from build123d import *

# Parameters (mm, degrees)
SKETCH2_W           = 304.8
SKETCH2_H           = 304.8
BOSS_EXTRUDE1_DEPTH = 15
SKETCH2_3_W         = 57
SKETCH2_3_H         = 3
SKETCH2_3_W_2       = 93.5
SKETCH2_3_W_3       = 130
SKETCH2_3_W_4       = 3
SKETCH2_3_H_2       = 16
SKETCH2_3_H_3       = 17.5
BOSS_EXTRUDE2_DEPTH = 17.5
CUT_EXTRUDE1_DEPTH  = 17.5
CUT_EXTRUDE2_DEPTH  = 17.5
CUT_EXTRUDE3_DEPTH  = 17.5
CUT_EXTRUDE4_DEPTH  = 17.5
CUT_EXTRUDE5_DEPTH  = 17.5
SKETCH2_5_R         = 2
BOSS_EXTRUDE3_DEPTH = 20
SKETCH8_W           = 20
SKETCH8_H           = 95
BOSS_EXTRUDE4_DEPTH = 45
CUT_EXTRUDE6_DEPTH  = 45
SKETCH11_W          = 12.681432754
SKETCH11_H          = 17.5
CUT_EXTRUDE8_DEPTH  = 35
SKETCH10_R          = 2
CUT_EXTRUDE7_DEPTH  = 45


with BuildPart() as part:
    # Sketch2 → Boss-Extrude1 (new body)
    with BuildSketch(Plane.XY):
        with Locations((152.4, 152.4)):
            Rectangle(SKETCH2_W, SKETCH2_H)
    extrude(amount=-BOSS_EXTRUDE1_DEPTH)

    # Sketch2_3 → Boss-Extrude2 (add)
    with BuildSketch(Plane.XY):
        Polygon((93.5, 282.8), (0, 282.8), (0, 279.8), (21.107831574, 279.8), (24.107831574, 279.8), (93.5, 279.8), align=None)
        with BuildLine():
            Line((40, 256.8), (40, 259.8))
            ThreePointArc((40, 259.8), (16.665476221, 250.134523779), (7, 226.8))
            Line((7, 226.8), (7, 180.8))
            Line((7, 180.8), (10, 180.8))
            Line((10, 180.8), (10, 226.8))
            ThreePointArc((10, 226.8), (18.786796564, 248.013203436), (40, 256.8))
        make_face()
        with Locations((65, 238.3)):
            Rectangle(SKETCH2_3_W, SKETCH2_3_H)
        with BuildLine():
            ThreePointArc((93.5, 302.8), (126.5, 269.8), (93.5, 236.8))
            Line((93.5, 236.8), (93.5, 239.8))
            ThreePointArc((93.5, 239.8), (123.5, 269.8), (93.5, 299.8))
            Line((93.5, 299.8), (93.5, 302.8))
        make_face()
        with Locations((46.75, 301.3)):
            Rectangle(SKETCH2_3_W_2, SKETCH2_3_H)
        with BuildLine():
            Line((7, 180.8), (10, 180.8))
            ThreePointArc((10, 180.8), (21.719007055, 152.507814231), (50.011192824, 140.788807176))
            Line((50.011192824, 140.788807176), (50.011192824, 137.788807176))
            ThreePointArc((50.011192824, 137.788807176), (19.597686711, 150.386493887), (7, 180.8))
        make_face()
        with Locations((115.011192824, 139.288807176)):
            Rectangle(SKETCH2_3_W_3, SKETCH2_3_H)
        with BuildLine():
            Line((180.011192824, 140.788807176), (180.011192824, 137.788807176))
            ThreePointArc((180.011192824, 137.788807176), (225.294551046, 153.531340693), (251.047093253, 193.969150516))
            Line((251.047093253, 193.969150516), (248.127809674, 194.660369283))
            ThreePointArc((248.127809674, 194.660369283), (223.433591119, 155.884387261), (180.011192824, 140.788807176))
        make_face()
        Polygon((252.275122275, 212.176070758), (255.194405854, 211.484851991), (251.047093253, 193.969150516), (248.127809674, 194.660369283), align=None)
        with BuildLine():
            ThreePointArc((281.424928951, 191.366981998), (283.869077464, 188.002900174), (284.733622888, 183.935533743))
            Line((284.733622888, 183.935533743), (284.733622888, 151.387820597))
            Line((284.733622888, 151.387820597), (281.733622888, 151.387820597))
            Line((281.733622888, 151.387820597), (281.733622888, 182.599847688))
            ThreePointArc((281.733622888, 182.599847688), (280.869077464, 186.667214118), (278.424928951, 190.031295942))
            Line((278.424928951, 190.031295942), (258.945596653, 207.570565524))
            Line((258.945596653, 207.570565524), (260.952988472, 209.8))
            Line((260.952988472, 209.8), (281.424928951, 191.366981998))
        make_face()
        Polygon((304.8, 124.8), (304.8, 279.8), (301.8, 279.8), (301.8, 148.186252327), (301.8, 133.38760374), (301.8, 124.8), align=None)
        with BuildLine():
            Line((301.8, 133.38760374), (301.8, 148.186252327))
            ThreePointArc((301.8, 148.186252327), (295.901436431, 128.741294171), (280.193920133, 115.850468689))
            Line((280.193920133, 115.850468689), (293.866088671, 121.513666325))
            ThreePointArc((293.866088671, 121.513666325), (298.395845267, 127.074583472), (301.8, 133.38760374))
        make_face()
        Polygon((287.505261485, 115.631748836), (304.8, 122.795464086), (304.8, 124.8), (301.8, 124.8), (293.866088671, 121.513666325), (280.193920133, 115.850468689), (257.453782439, 106.431195246), (260.952988472, 104.633437242), (284.733622888, 114.483698539), align=None)
        Polygon((263.8, 20), (263.8, 0), (304.8, 0), (304.8, 33), (301.8, 33), (301.8, 3), (266.8, 3), (266.8, 20), align=None)
        Polygon((91.199667441, 27.530149764), (92.438635381, 24.873174442), (89.266558126, 23.394010526), (86.547634765, 22.126155741), (83.375557511, 20.646991825), (82.126335472, 23.374526297), align=None)
        with Locations((22.607831574, 271.8)):
            Rectangle(SKETCH2_3_W_4, SKETCH2_3_H_2)
        with Locations((47.84178582, 228.05)):
            Rectangle(SKETCH2_3_W_4, SKETCH2_3_H_3)
        with Locations((114.353619172, 129.788807176)):
            Rectangle(SKETCH2_3_W_4, SKETCH2_3_H_2)
        Polygon((294.010879835, 99.925796783), (287.505261485, 115.631748836), (284.733622888, 114.483698539), (291.239241238, 98.777746486), align=None)
        Polygon((10.107831574, 4.345500571), (5, 16.3), (16, 21), (21.107831574, 9.045500571), align=None)
        Polygon((97.718923361, 5.267854785), (95, 4), (86.547634765, 22.126155741), (89.266558126, 23.394010526), align=None)
    extrude(amount=BOSS_EXTRUDE2_DEPTH)

    # Sketch3 → Cut-Extrude1 (cut)
    with BuildSketch(Plane(origin=(79.564500346, 37.101535829, 0), x_dir=(0, 0, 1), z_dir=(-0.906307787, -0.422618262, 0))):
        Polygon((17.5, -16.523503717), (0, -36.523503717), (17.5, -36.523503717), align=None)
    extrude(amount=-CUT_EXTRUDE1_DEPTH, mode=Mode.SUBTRACT)

    # Sketch4 → Cut-Extrude2 (cut)
    with BuildSketch(Plane(origin=(283.511449018, 117.434287271, 0), x_dir=(0, 0, 1), z_dir=(-0.923879533, -0.382683432, 0))):
        Polygon((17.5, -3.452640544), (0, -20.19369423), (17.5, -20.19369423), align=None)
    extrude(amount=-CUT_EXTRUDE2_DEPTH, mode=Mode.SUBTRACT)

    # Sketch5 → Cut-Extrude3 (cut)
    with BuildSketch(Plane.ZY.offset(-112.853619172)):
        Polygon((17.5, 137.788807176), (17.5, 121.788807176), (0, 121.788807176), align=None)
    extrude(amount=-CUT_EXTRUDE3_DEPTH, mode=Mode.SUBTRACT)

    # Sketch6 → Cut-Extrude4 (cut)
    with BuildSketch(Plane.ZY.offset(-46.34178582)):
        Polygon((17.5, 236.8), (17.5, 219.3), (0, 219.3), align=None)
    extrude(amount=-CUT_EXTRUDE4_DEPTH, mode=Mode.SUBTRACT)

    # Sketch7 → Cut-Extrude5 (cut)
    with BuildSketch(Plane.ZY.offset(-21.107831574)):
        Polygon((17.5, 279.8), (0, 263.8), (17.5, 263.8), align=None)
    extrude(amount=-CUT_EXTRUDE5_DEPTH, mode=Mode.SUBTRACT)

    # Sketch2_5 → Boss-Extrude3 (add)
    with BuildSketch(Plane.XY):
        with Locations((172.8, 55)):
            Circle(SKETCH2_5_R)
        with Locations((180.011192824, 210.788807176)):
            Circle(SKETCH2_5_R)
    extrude(amount=BOSS_EXTRUDE3_DEPTH)

    # Sketch8 → Boss-Extrude4 (add)
    with BuildSketch(Plane(origin=(0, 0, -15), x_dir=(-1, 0, 0), z_dir=(0, 0, -1))):
        with Locations((-152.4, 47.5)):
            Rectangle(SKETCH8_W, SKETCH8_H)
    extrude(amount=BOSS_EXTRUDE4_DEPTH)

    # Sketch9 → Cut-Extrude6 (cut)
    with BuildSketch(Plane(origin=(162.4, 0, 0), x_dir=(0, 0, -1), z_dir=(1, 0, 0))):
        Polygon((45.99140235, 95), (60, 95), (60, 0), align=None)
    extrude(amount=-CUT_EXTRUDE6_DEPTH, mode=Mode.SUBTRACT)

    # Sketch11 → Cut-Extrude8 (cut)
    with BuildSketch(Plane.XZ.offset(-279.8)):
        with Locations((6.340716377, 8.75)):
            Rectangle(SKETCH11_W, SKETCH11_H)
    extrude(amount=-CUT_EXTRUDE8_DEPTH, mode=Mode.SUBTRACT)

    # Sketch10 → Cut-Extrude7 (cut)
    with BuildSketch(Plane(origin=(10.11747851, 4.322922636, 0), x_dir=(0, 0, 1), z_dir=(-0.919576879, -0.392910121, 0))):
        with Locations((11, 6.524552525)):
            Circle(SKETCH10_R)
        with BuildLine():
            Line((17.5, 13.024552525), (11, 13.024552525))
            ThreePointArc((11, 13.024552525), (15.596194078, 11.120746603), (17.5, 6.524552525))
            Line((17.5, 6.524552525), (17.5, 13.024552525))
        make_face()
        with BuildLine():
            Line((17.5, 0.024552525), (17.5, 6.524552525))
            ThreePointArc((17.5, 6.524552525), (15.596194078, 1.928358447), (11, 0.024552525))
            Line((11, 0.024552525), (17.5, 0.024552525))
        make_face()
    extrude(amount=-CUT_EXTRUDE7_DEPTH, mode=Mode.SUBTRACT)


solid = part.part
CAD build for the part. Positions are in the model's coordinates, mm. A direction names the side the tool comes from. Round coordinates to 2 decimals unless told otherwise and drop trailing zeros. Write each loop counter-clockwise with the first axis right and the second up, starting at its lowest first coordinate (ties: lowest second). Pieces come first, ordered by that corner, then holes.
(1) Slice it at D-D, the plane y = 269.8. Write the cut outline in (x, z), and give its area (3 significant figures).
(2) 3-axis set-ups, long thin cutter, end or side, ignore diameter. For faces 1 (the face through (268.983, 111.207, 8.628)), 2 (the face through (88.955, 16.964, 4.739)), 3 (the face through (41, 236.8, 9)): which of +Z, -Z, +X, -X, +Y, -Y reach the whole face in a straight line?
(3) Slice it at A-A, the plane y = 89.5. Write the cut outline in (x, z).
(4) Drop flat-ended pins along their axis: P1, Ø9, axis at y = 198.5, z = 6, coming from the -X side; P2, Ø19, axis at y = 23, z = 5.5, coming from the -X side; P3, Ø0.9, axis at y = 281, z = 6, coming from the +X side; P4, Ø5, axis at x = 35, y = 135.5, coming from the -Z side. Give the stop position or say it passes through.
(5) Probe line 1 along Y through (x, z) = (77.5, 4); line 2 along X through (y, z) = (193, 9); line 3 along Z through (x, y) = (137.5, 55). List the from-to ranges inside material, lowest first.
(6) Slice it at B-B, the plane z = -36. Write the cut outline in (x, y), and give its area (3 significant figures).
(7) Mould opens along X. For faces 4 (the face through (81, 137.789, 9)), 5 (the face through (10, 203, 9)), 6 (the face through (0, 150, -7)), 7 (the face through (290.081, 109.414, 6.683)) say: pulls with the +X half, pulls with the -X half, needs draft (parallel to the pull), parting line crosses it, or undercut.
(8) Slice it at C-C, the plane y = 203. Write the cut outline in (x, z).
From the geometry:
1. outline: (0, -15) - (304.8, -15) - (304.8, 17.5) - (301.8, 17.5) - (301.8, 0) - (126.5, 0) - (126.5, 17.5) - (123.5, 17.5) - (123.5, 0) - (24.11, 0) - (24.11, 6.56) - (21.11, 6.56) - (21.11, 0) - (0, 0) - close
1. area: 4,700 mm2
2. face 1: +Z, -X
2. face 2: +Z, -Y
2. face 3: +Z
3. outline: (0, -15) - (142.4, -15) - (142.4, -46.8) - (162.4, -46.8) - (162.4, -15) - (304.8, -15) - (304.8, 0) - (0, 0) - close
4. P1: stops at x = 7
4. P2: stops at x = 0
4. P3: stops at x = 124.7
4. P4: stops at z = -15
5. line 1: y = 137.79 to 140.79, 236.8 to 239.8, 279.8 to 282.8, 299.8 to 302.8
5. line 2: x = 7 to 10, 247.71 to 250.81, 275.13 to 279.61, 301.8 to 304.8
5. line 3: z = -15 to 0
6. outline: (142.4, 0) - (162.4, 0) - (162.4, 95) - (142.4, 95) - close
6. area: 1,900 mm2
7. face 4: needs draft
7. face 5: undercut
7. face 6: pulls with the -X half
7. face 7: pulls with the +X half
8. outline: (0, -15) - (304.8, -15) - (304.8, 17.5) - (301.8, 17.5) - (301.8, 0) - (268.51, 0) - (268.51, 17.5) - (264.02, 17.5) - (264.02, 0) - (253.19, 0) - (253.19, 17.5) - (250.1, 17.5) - (250.1, 0) - (10, 0) - (10, 17.5) - (7, 17.5) - (7, 0) - (0, 0) - close
